Geometry check sheet. Reference: the model listing, model coordinates, mm. Face numbers are marked on the shaded views. A direction names the side the tool comes from. Round coordinates to 2 decimals unless told otherwise and drop trailing zeros. Write each loop counter-clockwise with the first axis right and the second up, starting at its lowest first coordinate (ties: lowest second). Pieces come first, ordered by that corner, then holes. Notation, with made-up numbers: (70.5, 46) - (74.5, 46) arc R17 cw to (74.5, 63) - close; hole circle Ø1 at (-33.75, 50). An arc over 180 degrees is marked (long way). Return JSON: item names as keys, results as strings. Group by question number.
from build123d import *

# Parameters (mm, degrees)
BOSS_EXTRUDE1_DEPTH = 83.0326
SKETCH2_W           = 61.8998
SKETCH2_H           = 21.463
BOSS_EXTRUDE2_DEPTH = 3.175
SKETCH3_W           = 25.4
SKETCH3_H           = 5.08
CUT_EXTRUDE1_DEPTH  = 107.886039958
FILLET1_R           = 0.762
FILLET2_R           = 0.762
FILLET3_R           = 0.762
SKETCH5_W           = 16.529901782
SKETCH5_H           = 9.525
CUT_EXTRUDE2_DEPTH  = 90.51870739
SKETCH42_W          = 25.4
SKETCH42_H          = 6.9088
CUT_EXTRUDE3_DEPTH  = 3.175


with BuildPart() as part:
    # Sketch1 → Boss-Extrude1 (new body)
    with BuildSketch(Plane(origin=(0, 0, 0), x_dir=(0, 0, -1), z_dir=(1, 0, 0))):
        Polygon((-27.7749, 9.525), (-24.0411, 9.525), (-24.0411, 12.7), (-30.9499, 12.7), (-30.9499, -3.175), (-30.9499, -8.763), (30.9499, -8.763), (30.9499, -3.175), (30.9499, 12.7), (24.0411, 12.7), (24.0411, 9.525), (27.7749, 9.525), (27.7749, 0), (-27.7749, 0), align=None)
    extrude(amount=BOSS_EXTRUDE1_DEPTH)

    # Sketch2 → Boss-Extrude2 (add)
    with BuildSketch(Plane(origin=(83.0326, 0, 0), x_dir=(0, 0, -1), z_dir=(1, 0, 0))):
        with Locations((0, 1.9685)):
            Rectangle(SKETCH2_W, SKETCH2_H)
    extrude(amount=BOSS_EXTRUDE2_DEPTH)

    # Sketch3 → Cut-Extrude1 (cut, through all)
    with BuildSketch(Plane.XY.offset(30.9499)):
        with Locations((24.0538, -4.815937668)):
            Rectangle(SKETCH3_W, SKETCH3_H)
        with Locations((62.1538, -4.815937668)):
            Rectangle(SKETCH3_W, SKETCH3_H)
    extrude(amount=-CUT_EXTRUDE1_DEPTH, mode=Mode.SUBTRACT)

    # Fillet1
    fillet1_edges = [part.edges().sort_by_distance(p)[0] for p in [
        (24.0538, -7.355937668, -30.9499),
        (24.0538, -7.355937668, 30.9499),
        (62.1538, -7.355937668, -30.9499),
        (62.1538, -7.355937668, 30.9499),
    ]]
    fillet(fillet1_edges, radius=FILLET1_R)

    # Fillet2
    fillet2_edges = [part.edges().sort_by_distance(p)[0] for p in [
        (11.3538, -5.196937668, -30.9499),
        (24.0538, -2.275937668, -30.9499),
        (36.7538, -5.196937668, -30.9499),
        (49.4538, -5.196937668, -30.9499),
        (62.1538, -2.275937668, -30.9499),
        (74.8538, -5.196937668, -30.9499),
    ]]
    fillet(fillet2_edges, radius=FILLET2_R)

    # Fillet3
    fillet3_edges = [part.edges().sort_by_distance(p)[0] for p in [
        (74.8538, -5.196937668, 30.9499),
        (62.1538, -2.275937668, 30.9499),
        (49.4538, -5.196937668, 30.9499),
        (11.3538, -5.196937668, 30.9499),
        (24.0538, -2.275937668, 30.9499),
        (36.7538, -5.196937668, 30.9499),
    ]]
    fillet(fillet3_edges, radius=FILLET3_R)

    # Sketch5 → Cut-Extrude2 (cut, through all)
    with BuildSketch(Plane.ZY.offset(-83.0326)):
        with Locations((0, 4.7625)):
            Rectangle(SKETCH5_W, SKETCH5_H)
    extrude(amount=-CUT_EXTRUDE2_DEPTH, mode=Mode.SUBTRACT)

    # Sketch42 → Cut-Extrude3 (cut)
    with BuildSketch(Plane(origin=(0, 12.7, 0), x_dir=(1, 0, 0), z_dir=(0, 1, 0))):
        with Locations((12.7, 27.4955)):
            Rectangle(SKETCH42_W, SKETCH42_H)
        with Locations((12.7, -27.4955)):
            Rectangle(SKETCH42_W, SKETCH42_H)
    extrude(amount=-CUT_EXTRUDE3_DEPTH, mode=Mode.SUBTRACT)


solid = part.part
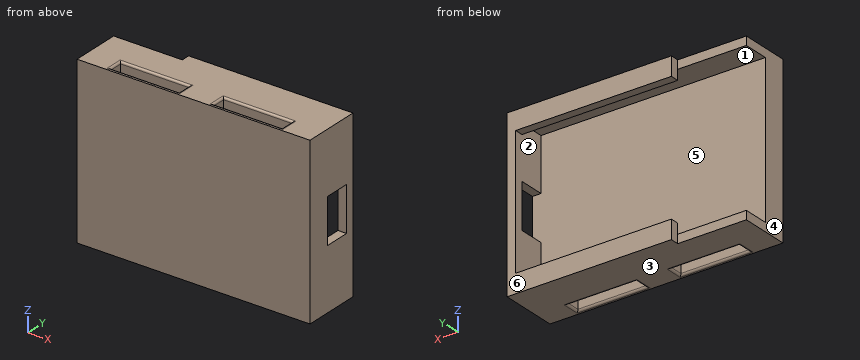
1. Section check A-A (x = 21). Enter the section's corners in (y, z) (3 decimals).
2. Section check C-C (y = -5). Enter the section's corners in (x, z), and give its area (3 significant figures).
3. Mould release check, pull along Z, two halves, no side actions. Record for the marked faces 1, 2, 3 and 4: pulls with the +Z half, pulls with the -Z half, needs draft (parallel to the pull), parting line crosses it, or undercut.
4. Material ranges on line 1 along X through (y, z) = (-5.75, 14); line 2 along Y through (x, z) = (66, 27) (3 decimals); line 3 along Y through (x, z) = (66.5, -2.5), recorded low to high.
5. Section check B-B (z = 0). Enter the section's corners in (x, y) (3 decimals).
6. Depth check by flat-ended pin: pin 1 Ø3.5 at (x, z) = (15, -30) entering from +Y (3 decimals); pin 2 Ø1 at (y, z) = (10.5, 26) entering from -X; pin 3 Ø3 at (x, z) = (76.5, 0.5) entering from +Y. Enter the tip coordinate at first touch or a pass-through.
7. Tool access check on the marked faces 5 and 6. Record the directions out of +Z, -Z, +X, -X, +Y, -Y that give a thin tool (end or side, any length) a straight path to the whole face; none if there is none.
8. Section check D-D (y = 8.5). Enter the section's corners in (x, z).
Result sheet:
{
 "1": {"outline": "(-8.763, -30.95) - (-8.118, -30.95) arc R0.762 ccw to (-7.356, -30.188) - (-7.356, 30.188) arc R0.762 ccw to (-8.118, 30.95) - (-8.763, 30.95) - close; (-2.276, -30.188) arc R0.762 ccw to (-1.514, -30.95) - (9.525, -30.95) - (9.525, -27.775) - (0, -27.775) - (0, 27.775) - (9.525, 27.775) - (9.525, 30.95) - (-1.514, 30.95) arc R0.762 ccw to (-2.276, 30.188) - close"},
 "2": {"outline": "(0, -30.95) - (10.59, -30.95) arc R0.76 ccw to (11.35, -30.19) - (11.35, 30.19) arc R0.76 ccw to (10.59, 30.95) - (0, 30.95) - close; (36.75, -30.19) arc R0.76 ccw to (37.52, -30.95) - (48.69, -30.95) arc R0.76 ccw to (49.45, -30.19) - (49.45, 30.19) arc R0.76 ccw to (48.69, 30.95) - (37.52, 30.95) arc R0.76 ccw to (36.75, 30.19) - close; (74.85, -30.19) arc R0.76 ccw to (75.62, -30.95) - (86.21, -30.95) - (86.21, 30.95) - (75.62, 30.95) arc R0.76 ccw to (74.85, 30.19) - close", "area": "2,190 mm²"},
 "3": {"face 1": "undercut", "face 2": "undercut", "face 3": "pulls with the -Z half", "face 4": "needs draft"},
 "4": {"line 1": "x = 0 to 11.35, 36.75 to 49.45, 74.85 to 86.21", "line 2": "y = -8.763 to -7.356, -2.276 to 0, 9.525 to 12.7", "line 3": "y = -8.76 to -7.36, -2.28 to 0"},
 "5": {"outline": "(0, -8.763) - (86.208, -8.763) - (86.208, 0) - (0, 0) - close; (83.033, 9.525) - (86.208, 9.525) - (86.208, 12.7) - (83.033, 12.7) - close; hole (11.354, -7.356) - (36.754, -7.356) - (36.754, -2.276) - (11.354, -2.276) - close; hole (49.454, -7.356) - (74.854, -7.356) - (74.854, -2.276) - (49.454, -2.276) - close"},
 "6": {"pin 1": "stops at y = 9.525", "pin 2": "stops at x = 25.4", "pin 3": "stops at y = 0"},
 "7": {"face 5": "-X", "face 6": "+Z, -Z, +X, -X, +Y"},
 "8": {"outline": "(0, -30.95) - (86.21, -30.95) - (86.21, -8.26) - (83.03, -8.26) - (83.03, -27.77) - (0, -27.77) - close; (0, 27.77) - (83.03, 27.77) - (83.03, 8.26) - (86.21, 8.26) - (86.21, 30.95) - (0, 30.95) - close"}
}
